The model under review builds one solid part; all positions refer to its coordinate system, in mm. A direction names the side the tool comes from. Round coordinates to 2 decimals unless told otherwise and drop trailing zeros. Write each loop counter-clockwise with the first axis right and the second up, starting at its lowest first coordinate (ties: lowest second). Pieces come first, ordered by that corner, then holes. Notation, with made-up numbers: M 87,67 L 135,67 A29 cw 135,102 Z; hole C -27,-2.75 d5. An arc over 180 degrees is marked long. One line per item, written item: value. Start each with the question number.
1) Take a section at C-C, the plane z = -6. Write out the cut boundary in (x, y).
2) Wall thickness on probe 1 along Z at (x, y) = (-27.5, 1.8); probe 2 along X at (y, z) = (2.4, -25); probe 3 along Z at (x, y) = (-27, 3): over which ranges is each line inside the solid? List them lowest first.
3) Take a section at D-D, the plane x = -24. Write out the cut boundary in (y, z), and give its area (3 significant figures).
4) For P1, Ø4, axis at x = -27.5, z = -25, coming from the -Y side; P2, Ø6, axis at x = -16, y = -26, coming from the +Z side; P3, Ø12, axis at x = 3, z = -5.5, coming from the -Y side, all flat-tipped, find the tip position at first contact; note any pin that passes through.
5) Tool access review of faces 1 (the face through (0, -27, -34)), 2 (the face through (23.35, -20.93, -36.96)): name each direction out of +Z, -Z, +X, -X, +Y, -Y from which nothing blocks a thin tool from reaching the whole face with its end or side.
6) Take a section at B-B, the plane y = -24.5. Write out the cut boundary in (x, z).
7) Mouldability with a two-part tool opening along X and no side actions: class faces 3 (the face through (-26.4, -19.8, -37)), 4 (the face through (-34, -10, -35)), 5 (the face through (-8, -25, -40)) as +X half, -X half, draft (parallel to the pull), parting line (faces both ways), or undercut.
8) Take a section at A-A, the plane x = 16. Write out the cut boundary in (y, z).
from build123d import *

# Parameters (mm, degrees)
SKETCH_1_W          = 68
SKETCH_1_H          = 40
SKETCH_1_R          = 2.5
EXTRUDE_1_DEPTH     = 6
SKETCH_3_W          = 68
SKETCH_3_H          = 6
EXTRUDE_2_DEPTH     = 50
CUT_EXTRUDE_1_REACH = 8
SKETCH_4_R          = 8
SKETCH_4_R_2        = 3
SKETCH_5_R          = 3.3
CUT_EXTRUDE_2_DEPTH = 10


with BuildPart() as part:
    # 草图1 → 凸台-拉伸1 (new body)
    with BuildSketch(Plane(origin=(0, 0, 0), x_dir=(1, 0, 0), z_dir=(0, 1, 0))):
        with Locations((0, 20)):
            Rectangle(SKETCH_1_W, SKETCH_1_H)
        with Locations((-27.5, 25)):
            Circle(SKETCH_1_R, mode=Mode.SUBTRACT)
        with Locations((27.5, 25)):
            Circle(SKETCH_1_R, mode=Mode.SUBTRACT)
        with Locations((-27.5, 5)):
            Circle(SKETCH_1_R, mode=Mode.SUBTRACT)
    extrude(amount=EXTRUDE_1_DEPTH)

    # 草图3 → 凸台-拉伸2 (add)
    with BuildSketch(Plane(origin=(0, 6, 0), x_dir=(1, 0, 0), z_dir=(0, 1, 0))):
        with Locations((0, 37)):
            Rectangle(SKETCH_3_W, SKETCH_3_H)
    extrude(amount=-EXTRUDE_2_DEPTH)

    # 草图4 → 切除-拉伸1 (cut, up to next)
    with BuildSketch(Plane.XY.offset(-34), mode=Mode.PRIVATE) as cut_extrude_1_sk1:
        with Locations((0, -18)):
            Circle(SKETCH_4_R)
    cut_extrude_1_tool1 = extrude(cut_extrude_1_sk1.sketch, amount=-CUT_EXTRUDE_1_REACH, mode=Mode.PRIVATE) & part.part
    add(cut_extrude_1_tool1.solids().sort_by_distance((0, -18, -34))[0], mode=Mode.SUBTRACT)
    # 草图4 → 切除-拉伸1 (cut, up to next)
    with BuildSketch(Plane.XY.offset(-34), mode=Mode.PRIVATE) as cut_extrude_1_sk2:
        with Locations((24, -18)):
            Circle(SKETCH_4_R_2)
    cut_extrude_1_tool2 = extrude(cut_extrude_1_sk2.sketch, amount=-CUT_EXTRUDE_1_REACH, mode=Mode.PRIVATE) & part.part
    add(cut_extrude_1_tool2.solids().sort_by_distance((24, -18, -34))[0], mode=Mode.SUBTRACT)
    # 草图4 → 切除-拉伸1 (cut, up to next)
    with BuildSketch(Plane.XY.offset(-34), mode=Mode.PRIVATE) as cut_extrude_1_sk3:
        with Locations((-24, -18)):
            Circle(SKETCH_4_R_2)
    cut_extrude_1_tool3 = extrude(cut_extrude_1_sk3.sketch, amount=-CUT_EXTRUDE_1_REACH, mode=Mode.PRIVATE) & part.part
    add(cut_extrude_1_tool3.solids().sort_by_distance((-24, -18, -34))[0], mode=Mode.SUBTRACT)

    # 草图5 → 切除-拉伸2 (cut)
    with BuildSketch(Plane.XZ):
        with Locations((15.999999998, -6)):
            Circle(SKETCH_5_R)
    extrude(amount=-CUT_EXTRUDE_2_DEPTH, mode=Mode.SUBTRACT)


solid = part.part
Checked values:
1. outline: M -34,0 L -29.79,0 L -29.79,6 L -34,6 Z; M -25.21,0 L 12.7,0 L 12.7,6 L -25.21,6 Z; M 19.3,0 L 34,0 L 34,6 L 19.3,6 Z
2. probe 1: z = -40 to -27.5, -22.5 to -7.5, -2.5 to 0
2. probe 2: x = -34 to -30, -25 to 25, 30 to 34
2. probe 3: z = -40 to -27.45, -22.55 to -7.45, -2.55 to 0
3. outline: M -44,-40 L -21,-40 L -21,-34 L -44,-34 Z; M -15,-40 L 6,-40 L 6,0 L 0,0 L 0,-34 L -15,-34 Z
3. area: 468 mm2
4. P1: passes through
4. P2: stops at z = -34
4. P3: stops at y = 0
5. face 1: +Z, +X, -X, -Y
5. face 2: +Z, -Z
6. outline: M -34,-40 L -4.66,-40 L -4.66,-34 L -34,-34 Z; M 4.66,-40 L 34,-40 L 34,-34 L 4.66,-34 Z
7. face 3: undercut
7. face 4: -X half
7. face 5: draft
8. outline: M -44,-40 L 6,-40 L 6,-9.3 L 0,-9.3 L 0,-34 L -44,-34 Z; M 0,-2.7 L 6,-2.7 L 6,0 L 0,0 Z
